Verification items for the finished model (mm, model axes). A direction names the side the tool comes from. Give positions to 0.01 mm unless a question says otherwise; leave off trailing zeros. Loops run counter-clockwise (first coordinate to the right, second up) from the corner with the lowest first, then second, coordinate; pieces in that order, holes last. Notation, with made-up numbers: M -10.75,74 L 32.25,74 A10 cw 32.25,85 Z; hole C 43.25,-11.5 d2. An arc over 180 degrees is marked long. Answer in a Markdown table with one row per item.
```python
from build123d import *

# Parameters (mm, degrees)
MODEL_R             = 7.5
BOSS_EXTRUDE1_DEPTH = 3


with BuildPart() as part:
    # Model → Boss-Extrude1 (new body)
    with BuildSketch(Plane.XY):
        Polygon((21, -151.199653678), (18, -151.199653678), (18, -148.199653678), (21, -148.199653678), (21, -142.699653678), (24, -142.699653678), (24, -148.199653678), (27, -148.199653678), (27, -151.199653678), (24, -151.199653678), (24, -156.199653678), (30, -156.199653678), (30, -159.199653678), (40, -159.199653678), (40, -156.199653678), (54.9, -156.199653678), (54.9, -159.199653678), (64.9, -159.199653678), (64.9, -156.199653678), (70.9, -156.199653678), (70.9, -151.199653678), (67.9, -151.199653678), (67.9, -148.199653678), (70.9, -148.199653678), (70.9, -142.699653678), (73.9, -142.699653678), (73.9, -148.199653678), (76.9, -148.199653678), (76.9, -151.199653678), (73.9, -151.199653678), (73.9, -156.199653678), (79.9, -156.199653678), (79.9, -159.199653678), (89.9, -159.199653678), (89.9, -156.199653678), (92.9, -156.199653678), (92.9, -136.199653678), (89.9, -136.199653678), (89.9, -116.199653678), (92.9, -116.199653678), (92.9, -96.199653678), (89.9, -96.199653678), (89.9, -93.199653678), (79.9, -93.199653678), (79.9, -96.199653678), (73.9, -96.199653678), (73.9, -101.199653678), (76.9, -101.199653678), (76.9, -104.196392179), (73.9, -104.196392179), (73.9, -109.196392179), (70.9, -109.196392179), (70.9, -104.196392179), (67.9, -104.196392179), (67.9, -101.199653678), (70.9, -101.199653678), (70.9, -96.199653678), (64.9, -96.199653678), (64.9, -93.199653678), (54.9, -93.199653678), (54.9, -96.199653678), (40, -96.199653678), (40, -93.199653678), (30, -93.199653678), (30, -96.199653678), (24, -96.199653678), (24, -101.199653678), (27, -101.199653678), (27, -104.196392179), (24, -104.196392179), (24, -109.196392179), (21, -109.196392179), (21, -104.196392179), (18, -104.196392179), (18, -101.199653678), (21, -101.199653678), (21, -96.199653678), (15, -96.199653678), (15, -93.199653678), (5, -93.199653678), (5, -96.199653678), (2, -96.199653678), (2, -116.199653678), (5, -116.199653678), (5, -136.199653678), (2, -136.199653678), (2, -156.199653678), (5, -156.199653678), (5, -159.199653678), (15, -159.199653678), (15, -156.199653678), (21, -156.199653678), align=None)
        with Locations((17, -122.199653678)):
            Circle(MODEL_R, mode=Mode.SUBTRACT)
    extrude(amount=BOSS_EXTRUDE1_DEPTH)


solid = part.part
```
Item 1: Go/stop test with flat-tipped pins: pin 1 (0.9 mm diameter, centred on y = -158.5, z = 1, fed in from +X); pin 2 (0.9 mm diameter, centred on y = -94.5, z = 2, fed in from -X); pin 3 (1.5 mm diameter, centred on x = 69, z = 1, fed in from +Y). Record where each tip stops, or that it passes through.
Reported:
| item | result |
|---|---|
| pin 1 | stops at x = 89.9 |
| pin 2 | stops at x = 5 |
| pin 3 | stops at y = -96.2 |
Item 2: Tool access check on faces 1 (the flat face through (75, -148.2, 1)), 2 (the flat face through (70.9, -99, 1)), 3 (the flat face through (70.9, -145, 1)), 4 (the flat face through (3, -156.2, 1)). Record the directions out of +Z, -Z, +X, -X, +Y, -Y that give a thin tool (end or side, any length) a straight path to the whole face; none if there is none.
Reported:
| item | result |
|---|---|
| face 1 | +Z, -Z |
| face 2 | +Z, -Z, +Y |
| face 3 | +Z, -Z, -Y |
| face 4 | +Z, -Z, -X, -Y |
Item 3: Sectioned sample at C-C (y = -117.5). Record the cut outline in (x, z).
Reported:
| item | result |
|---|---|
| outline | M 5,0 L 11.16,0 L 11.16,3 L 5,3 Z; M 22.84,0 L 89.9,0 L 89.9,3 L 22.84,3 Z |
Item 4: Sectioned sample at B-B (x = 17). Record the cut outline in (y, z).
Reported:
| item | result |
|---|---|
| outline | M -156.2,0 L -129.7,0 L -129.7,3 L -156.2,3 Z; M -114.7,0 L -96.2,0 L -96.2,3 L -114.7,3 Z |
Item 5: Release check for a two-part mould opening along X. For faces 5 (the flat face through (2, -146, 1)), 6 (the flat face through (60, -159.2, 1)), 7 (the flat face through (75, -104.196, 1)) record: released by +X, released by -X, zero draft, split by the parting line, or undercut.
Reported:
| item | result |
|---|---|
| face 5 | released by -X |
| face 6 | zero draft |
| face 7 | undercut |
Item 6: Scan lines: L1, parallel to Y at x = 76.5, z = 0.45; L2, parallel to Y at x = 17, z = 1.1; L3, parallel to X at y = -143, z = 0.7. Record each from-to range of solid material in increasing order. Write a range as [from, to].
Reported:
| item | result |
|---|---|
| L1 | y = [-156.2, -151.2], [-148.2, -104.2], [-101.2, -96.2] |
| L2 | y = [-156.2, -129.7], [-114.7, -96.2] |
| L3 | x = [2, 21], [24, 70.9], [73.9, 92.9] |
Item 7: Sectioned sample at D-D (x = 54). Record the cut outline in (y, z), and give its area (3 significant figures).
Reported:
| item | result |
|---|---|
| outline | M -156.2,0 L -96.2,0 L -96.2,3 L -156.2,3 Z |
| area | 180 mm^2 |
Item 8: Sectioned sample at A-A (y = -107). Record the cut outline in (x, z).
Reported:
| item | result |
|---|---|
| outline | M 2,0 L 21,0 L 21,3 L 2,3 Z; M 24,0 L 70.9,0 L 70.9,3 L 24,3 Z; M 73.9,0 L 92.9,0 L 92.9,3 L 73.9,3 Z |
